Verification items for the finished model (mm, model axes). Face numbers are marked on the shaded views. Coordinates: 2 decimals unless noted, no trailing zeros. Loops run counter-clockwise (first coordinate to the right, second up) from the corner with the lowest first, then second, coordinate; pieces in that order, holes last.
Q1. Material ranges on probe 1 along Z at (x, y) = (-30, 6.2); probe 2 along Z at (x, y) = (-30, 1.2); probe 3 along X at (y, z) = (6.5, -11.75), recorded low to high.
Q2. Sectioned sample at C-C (z = -10). Count the separate pieces of the cut face and the enclosed holes in it, then the cut area to 3 significant figures.
Q3. Sectioned sample at A-A (z = 0). Enter the section's corners in (x, y), then the cut area to 3 significant figures.
Q4. Sectioned sample at B-B (x = -30). Enter the section's corners in (y, z), then the cut area to 3 significant figures.
Q5. Go/stop test with flat-tipped pins: P1, Ø6.5, axis at x = 30.5, z = 9, coming from the +Y side; P2, Ø5.5, axis at x = 30, z = 10, coming from the -Y side; P3, Ø3, axis at x = -8, z = 2, coming from the -Y side; P4, Ø3, axis at x = -30, z = 10.5, coming from the +Y side. Record where each tip stops, or that it passes through.
Q6. Mould release check, pull along X, two halves, no side actions. Record for the marked faces 1, 2 and 3: +X half, -X half, draft (parallel to the pull), parting line (faces both ways), or undercut.
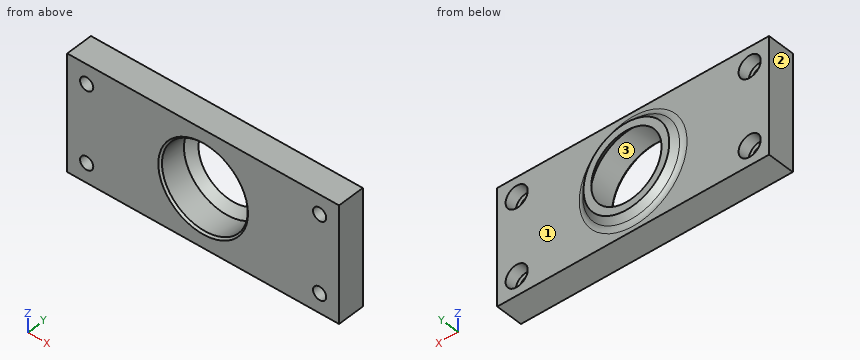
```python
from build123d import *

# Parameters (mm, degrees)
SKETCH1_R           = 15
SKETCH1_R_2         = 11.05
BOSS_EXTRUDE1_DEPTH = 7
BOSS_EXTRUDE2_DEPTH = 7
SKETCH3_R           = 1.7
CUT_EXTRUDE1_DEPTH  = 8
SKETCH4_R           = 2.85
CUT_EXTRUDE2_DEPTH  = 3
FILLET2_R           = 2
CHAMFER1_SIZE       = 0.5


with BuildPart() as part:
    # Sketch1 → Boss-Extrude1 (new body)
    with BuildSketch(Plane(origin=(0, 0, 0), x_dir=(1, 0, 0), z_dir=(0, 1, 0))):
        Circle(SKETCH1_R)
        Circle(SKETCH1_R_2, mode=Mode.SUBTRACT)
    extrude(amount=BOSS_EXTRUDE1_DEPTH)

    # Sketch2 → Boss-Extrude2 (add)
    with BuildSketch(Plane(origin=(0, 7, 0), x_dir=(1, 0, 0), z_dir=(0, 1, 0))):
        with BuildLine():
            Line((0, -15), (-35, -15))
            Line((-35, -15), (-35, 15))
            Line((-35, 15), (0, 15))
            ThreePointArc((0, 15), (-15, 0), (0, -15))
        make_face()
    boss_extrude2 = extrude(amount=-BOSS_EXTRUDE2_DEPTH)

    # Sketch3 → Cut-Extrude1 (cut, through all)
    with BuildSketch(Plane(origin=(0, 7, 0), x_dir=(1, 0, 0), z_dir=(0, 1, 0))):
        with Locations((-30, 10)):
            Circle(SKETCH3_R)
        with Locations((-30, -10)):
            Circle(SKETCH3_R)
    cut_extrude1 = extrude(amount=-CUT_EXTRUDE1_DEPTH, mode=Mode.SUBTRACT)

    # Sketch4 → Cut-Extrude2 (cut)
    with BuildSketch(Plane(origin=(0, 7, 0), x_dir=(1, 0, 0), z_dir=(0, 1, 0))):
        with Locations((-30, 10)):
            Circle(SKETCH4_R)
        with Locations((-30, -10)):
            Circle(SKETCH4_R)
    cut_extrude2 = extrude(amount=-CUT_EXTRUDE2_DEPTH, mode=Mode.SUBTRACT)

    # Mirror1: Boss-Extrude2, Cut-Extrude1, Cut-Extrude2 across plane
    add(boss_extrude2.mirror(Plane(origin=(0, 0, 0), x_dir=(0, 0, 1), z_dir=(1, 0, 0))))
    add(cut_extrude1.mirror(Plane(origin=(0, 0, 0), x_dir=(0, 0, 1), z_dir=(1, 0, 0))), mode=Mode.SUBTRACT)
    add(cut_extrude2.mirror(Plane(origin=(0, 0, 0), x_dir=(0, 0, 1), z_dir=(1, 0, 0))), mode=Mode.SUBTRACT)

    # Sketch6 → Revolve1 (revolve)
    with BuildSketch(Plane.XY):
        Polygon((11.05, 7), (9.05, 9), (11.05, 9), (13.05, 7), align=None)
    revolve(axis=Axis((0, 7, 0), (0, -1, 0)))

    # Fillet2
    fillet2_edges = [part.edges().sort_by_distance(p)[0] for p in [
        (-13.05, 7, 0),
    ]]
    fillet(fillet2_edges, radius=FILLET2_R)

    # Chamfer1
    chamfer1_edges = [part.edges().sort_by_distance(p)[0] for p in [
        (-11.05, 0, 0),
    ]]
    chamfer(chamfer1_edges, length=CHAMFER1_SIZE)


solid = part.part
```
Geometry check:
1. probe 1: z = -15 to -12.85, -7.15 to 7.15, 12.85 to 15
1. probe 2: z = -15 to -11.7, -8.3 to 8.3, 11.7 to 15
1. probe 3: x = -35 to -32.25, -27.75 to 27.75, 32.25 to 35
2. separate pieces: 3
2. enclosed holes: 0
2. area: 383 mm2
3. outline: (-35, 0) - (-11.55, 0) - (-11.05, 0.5) - (-11.05, 7) - (-9.05, 9) - (-11.05, 9) - (-12.46, 7.59) arc R2 cw to (-13.88, 7) - (-35, 7) - close; (9.05, 9) - (11.05, 7) - (11.05, 0.5) - (11.55, 0) - (35, 0) - (35, 7) - (13.88, 7) arc R2 cw to (12.46, 7.59) - (11.05, 9) - close
3. area: 343 mm2
4. outline: (0, -15) - (7, -15) - (7, -12.85) - (4, -12.85) - (4, -11.7) - (0, -11.7) - close; (0, -8.3) - (4, -8.3) - (4, -7.15) - (7, -7.15) - (7, 7.15) - (4, 7.15) - (4, 8.3) - (0, 8.3) - close; (0, 11.7) - (4, 11.7) - (4, 12.85) - (7, 12.85) - (7, 15) - (0, 15) - close
4. area: 149 mm2
5. P1: stops at y = 7
5. P2: stops at y = 0
5. P3: stops at y = 8.3
5. P4: stops at y = 4
6. face 1: draft
6. face 2: -X half
6. face 3: undercut
